Verification items for the finished model (mm, model axes). Face numbers are marked on the shaded views. Give positions to 0.01 mm unless a question says otherwise; leave off trailing zeros. Order: outer loops, then holes, each group sorted by start corner. A loop starts at its lowest first (then second) coordinate and runs counter-clockwise, first axis right, second up.
Autodesk Fusion 360 part; units mm, degrees
sketch "Schizzo1" plane through (0, 0, 0) normal (0, 0, 1) x (1, 0, 0)
  line L0 (50, 150) -> (168.7, 150) construction
  line L1 (168.7, 150) -> (168.7, 89.3) construction
  line L2 (168.7, 89.3) -> (50, 89.3) construction
  line L3 (50, 89.3) -> (50, 150) construction
  line L4 (50, 119.65) -> (168.7, 119.65) construction
  line L5 (109.35, 150) -> (109.35, 89.3) construction
  line L6 (168.6, 89.4) -> (50.1, 89.4)
  line L7 (50.1, 89.4) -> (50.1, 149.9)
  line L8 (50.1, 149.9) -> (168.6, 149.9)
  line L9 (168.6, 149.9) -> (168.6, 89.4)
  line L10 (168.6, 89.4) -> (50.1, 149.9) construction
  line L11 (50.1, 89.4) -> (168.6, 149.9) construction
  point P0 (109.35, 119.65)
  dimension "d1" = 118.7
  dimension "d2" = 60.7
  dimension "d3" = 0.1
  dimension "d4" = 0.1
extrude "Estrusione1" add sketch "Schizzo1" along normal blind 4
fillet "Raccordo1" radius 3 4 edges at (50.1, 89.4, 2) (168.6, 89.4, 2) (50.1, 149.9, 2) (168.6, 149.9, 2)
sketch "Schizzo2" plane through (0, 0, 4) normal (0, 0, 1) x (-1, 0, 0)
  arc A0 (-168.6, -146.9) -> (-165.6, -149.9) centre (-165.6, -146.9) ccw
  line L0 (-165.6, -149.9) -> (-53.1, -149.9)
  arc A1 (-53.1, -149.9) -> (-50.1, -146.9) centre (-53.1, -146.9) ccw
  line L1 (-50.1, -146.9) -> (-50.1, -92.4)
  arc A2 (-50.1, -92.4) -> (-53.1, -89.4) centre (-53.1, -92.4) ccw
  line L2 (-53.1, -89.4) -> (-165.6, -89.4)
  arc A3 (-165.6, -89.4) -> (-168.6, -92.4) centre (-165.6, -92.4) ccw
  line L3 (-168.6, -92.4) -> (-168.6, -146.9)
  line L4 (-50.1, -149.9) -> (-168.6, -149.9) construction
  line L5 (-168.6, -149.9) -> (-168.6, -89.4) construction
  line L6 (-168.6, -89.4) -> (-50.1, -89.4) construction
  line L7 (-50.1, -89.4) -> (-50.1, -149.9) construction
  line L8 (-50.1, -119.65) -> (-168.6, -119.65) construction
  line L9 (-109.35, -149.9) -> (-109.35, -89.4) construction
  line L10 (-166.6, -91.4) -> (-52.1, -91.4)
  line L11 (-52.1, -91.4) -> (-52.1, -147.9)
  line L12 (-52.1, -147.9) -> (-166.6, -147.9)
  line L13 (-166.6, -147.9) -> (-166.6, -91.4)
  line L14 (-166.6, -91.4) -> (-52.1, -147.9) construction
  line L15 (-52.1, -91.4) -> (-166.6, -147.9) construction
  line L16 (-70.6, -91.4) -> (-70.6, -147.9)
  line L17 (-63.6, -147.9) -> (-63.6, -91.4)
  line L18 (-52.1, -121.9) -> (-52.1, -147.9)
  line L19 (-103.6, -147.9) -> (-103.6, -91.4)
  line L20 (-110.6, -147.9) -> (-110.6, -91.4)
  line L21 (-143.6, -147.9) -> (-143.6, -91.4)
  line L22 (-150.6, -147.9) -> (-150.6, -91.4)
  line L23 (-52.1, -91.4) -> (-62.1, -91.4)
  line L24 (-62.1, -91.4) -> (-62.1, -117.4)
  line L25 (-62.1, -117.4) -> (-52.1, -117.4)
  line L26 (-52.1, -117.4) -> (-52.1, -91.4)
  line L27 (-102.1, -117.4) -> (-92.1, -117.4)
  line L28 (-92.1, -117.4) -> (-92.1, -91.4)
  line L29 (-102.1, -91.4) -> (-102.1, -117.4)
  line L30 (-92.1, -91.4) -> (-102.1, -91.4)
  line L31 (-142.1, -117.4) -> (-132.1, -117.4)
  line L32 (-132.1, -117.4) -> (-132.1, -91.4)
  line L33 (-142.1, -91.4) -> (-142.1, -117.4)
  line L34 (-132.1, -91.4) -> (-142.1, -91.4)
  line L35 (-52.1, -117.4) -> (-166.6, -117.4)
  line L36 (-52.1, -121.9) -> (-166.6, -121.9)
  point P0 (-109.35, -119.65)
  point P1 (-109.35, -119.65)
  dimension "d11" = 7
  dimension "d20" = 7
  dimension "d25" = 7
  dimension "d36" = 13.5
  dimension "d37" = 53.5
  dimension "d38" = 93.5
  dimension "d39" = 10
  dimension "d40" = 26
  dimension "d41" = 2
  dimension "d42" = 2
  dimension "d45" = -40
  dimension "d46" = 0
extrude "Estrusione2" cut sketch "Schizzo2" against normal blind 3 contours L10 L13 L22 L35 | L10 L21 L33 L35 | L12 L13 L22 L36 | L10 L31 L32 L33 L34 L35 | L10 L20 L32 L35 | L12 L20 L21 L36 | L10 L19 L29 L35 | L12 L16 L19 L36 | L10 L27 L28 L29 L30 L35 | L10 L16 L28 L35 | L11 L12 L17 L18 L36 | L10 L17 L24 L35 | L10 L11 L23 L24 L25 L26 L35
extrude "Estrusione3" cut sketch "Schizzo2" against normal blind 4 contours L10 L31 L32 L33 L34 L35 | L10 L27 L28 L29 L30 L35 | L10 L11 L23 L24 L25 L26 L35
ref_plane "Piano di lavoro1" through (109.35, 119.65, 4) normal (0, -1, 0) x (1, 0, 0)
sketch "Schizzo3" plane through (0, 119.65, 0) normal (0, -1, 0) x (-1, 0, 0)
  line L0 (-50.1, -4) -> (-168.7, -4) construction
  line L1 (-168.7, -4) -> (-168.7, 0) construction
  line L2 (-168.7, 0) -> (-50.1, 0) construction
  line L3 (-50.1, 0) -> (-50.1, -4) construction
  line L4 (-168.6, -4) -> (-50.1, -4) construction
  line L5 (-50.1, -1) -> (-168.7, -1) construction
  line L6 (-63.6, -4) -> (-63.6, 0) construction
  line L7 (-70.6, -4) -> (-70.6, 0) construction
  line L8 (-63.6, -4) -> (-63.6, -1) construction
  line L9 (-70.6, -4) -> (-70.6, -1) construction
  line L10 (-103.6, -4) -> (-103.6, 0) construction
  line L11 (-110.6, -4) -> (-110.6, 0) construction
  line L12 (-103.6, -4) -> (-103.6, -1) construction
  line L13 (-110.6, -4) -> (-110.6, -1) construction
  line L14 (-143.6, -4) -> (-143.6, 0) construction
  line L15 (-150.6, -4) -> (-150.6, 0) construction
  line L16 (-143.6, -4) -> (-143.6, -1) construction
  line L17 (-150.6, -4) -> (-150.6, -1) construction
  line L18 (-63.6, -4) -> (-65.3321, -1)
  line L19 (-63.6, -4) -> (-60.1359, -4) construction
  line L20 (-70.6, -4) -> (-68.8679, -1)
  line L21 (-70.6, -4) -> (-67.1359, -4) construction
  line L22 (-63.6, -4) -> (-63.6, -1)
  line L23 (-63.6, -1) -> (-65.3321, -1)
  line L24 (-68.8679, -1) -> (-70.6, -1)
  line L25 (-70.6, -1) -> (-70.6, -4)
  line L26 (-103.6, -1) -> (-103.6, -4)
  line L27 (-103.6, -4) -> (-105.3321, -1)
  line L28 (-105.3321, -1) -> (-103.6, -1)
  line L29 (-110.6, -1) -> (-110.6, -4)
  line L30 (-110.6, -4) -> (-108.8679, -1)
  line L31 (-108.8679, -1) -> (-110.6, -1)
  line L32 (-143.6, -1) -> (-143.6, -4)
  line L33 (-143.6, -4) -> (-145.3321, -1)
  line L34 (-145.3321, -1) -> (-143.6, -1)
  line L35 (-150.6, -1) -> (-150.6, -4)
  line L36 (-150.6, -4) -> (-148.8679, -1)
  line L37 (-148.8679, -1) -> (-150.6, -1)
  line L38 (-110.6, -1) -> (-143.6, -1)
  point P0 (-168.7, 0)
  dimension "d28" = 120
  dimension "d29" = 60
  dimension "d30" = 30
  dimension "d31" = 30
  dimension "d32" = 30
  dimension "d33" = 30
extrude "Estrusione4" cut sketch "Schizzo3" along normal blind 25 from surface at 2.5
extrude "Estrusione6" cut sketch "Schizzo3" against normal blind 25 from surface at -2.5
sketch "Schizzo4" plane through (0, 0, 4) normal (0, 0, 1) x (-1, 0, 0)
  line L0 (-50.1, -149.9) -> (-168.6, -149.9) construction
  line L1 (-168.6, -149.9) -> (-168.6, -89.4) construction
  line L2 (-168.6, -89.4) -> (-50.1, -89.4) construction
  line L3 (-50.1, -89.4) -> (-50.1, -149.9) construction
  line L4 (-165.6, -149.9) -> (-53.1, -149.9) construction
  line L5 (-53.1, -89.4) -> (-165.6, -89.4) construction
  line L6 (-50.1, -146.9) -> (-50.1, -92.4) construction
  line L7 (-168.6, -92.4) -> (-168.6, -146.9) construction
  line L8 (-50.1, -149.9) -> (-168.6, -149.9)
  line L9 (-168.6, -149.9) -> (-168.6, -147.9)
  line L10 (-168.6, -147.9) -> (-50.1, -147.9)
  line L11 (-50.1, -147.9) -> (-50.1, -149.9)
  line L12 (-50.1, -89.4) -> (-168.6, -89.4)
  line L13 (-168.6, -89.4) -> (-168.6, -91.4)
  line L14 (-168.6, -91.4) -> (-50.1, -91.4)
  line L15 (-50.1, -91.4) -> (-50.1, -89.4)
  dimension "d51" = 2
  dimension "d52" = 2
extrude "Estrusione5" cut sketch "Schizzo4" against normal blind 2
equation "d28 = 90 deg + 30 deg"
equation "d52 = d51"
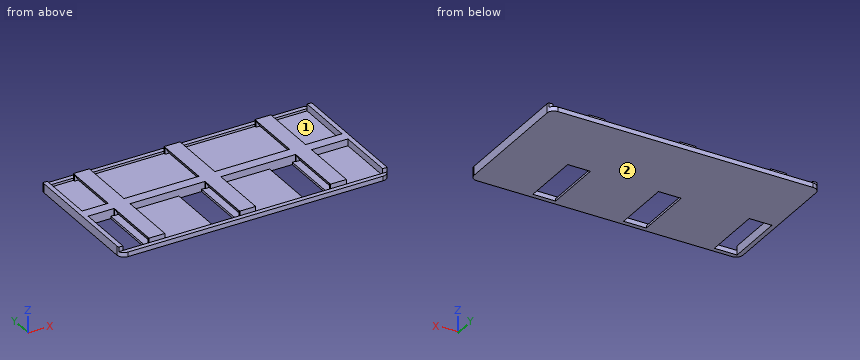
(1) Section check B-B, the plane x = 101. Enter the section's corners in (y, z), then the cut area to 3 significant figures.
Solved:
outline: (89.4, 0) - (91.4, 0) - (91.4, 2) - (89.4, 2) - close; (117.4, 0) - (149.9, 0) - (149.9, 2) - (147.9, 2) - (147.9, 1) - (121.9, 1) - (121.9, 4) - (117.4, 4) - close
area: 52.0 mm2
(2) Scan lines: line 1 (X direction, y = 111, z = 0.35); line 2 (Y direction, x = 70.5, z = 2.6); line 3 (X direction, y = 92, z = 2.1). Record each from-to range of solid material in increasing order.
Solved:
line 1: x = 50.1 to 52.1, 62.1 to 92.1, 102.1 to 132.1, 142.1 to 168.6
line 2: y = 91.4 to 92.15, 117.15 to 122.15, 147.15 to 147.9
line 3: x = 50.13 to 52.1, 63.6 to 70.6, 103.6 to 110.6, 143.6 to 150.6, 166.6 to 168.57
(3) Go/stop test with flat-tipped pins: pin 1 (0.5 mm diameter, centred on x = 150, z = 3, fed in from +Y); pin 2 (1.5 mm diameter, centred on x = 167.5, z = 3.5, fed in from -Y); pin 3 (1.5 mm diameter, centred on x = 62.5, y = 130.5, fed in from +Z). Record where each tip stops, or that it passes through.
Solved:
pin 1: stops at y = 147.9
pin 2: stops at y = 91.4
pin 3: stops at z = 1
(4) Release check for a two-part mould opening along X. For the marked faces 1 and 2 record: pulls with the +X half, pulls with the -X half, needs draft (parallel to the pull), parting line crosses it, or undercut.
Solved:
face 1: undercut
face 2: needs draft
(5) Section check D-D, the plane x = 67. Enter the section's corners in (y, z).
Solved:
outline: (89.4, 0) - (149.9, 0) - (149.9, 2) - (147.9, 2) - (147.9, 4) - (91.4, 4) - (91.4, 2) - (89.4, 2) - close
(6) Section check A-A, the plane y = 115.5. Give the number of separate pieces and of enclosed holes in the cut face, then the cut area to 3 significant figures.
Solved:
separate pieces: 4
enclosed holes: 0
area: 148 mm2
(7) Section check C-C, the plane y = 140. Enter the section's corners in (x, z), then the cut area to 3 significant figures.
Solved:
outline: (50.1, 0) - (168.6, 0) - (168.6, 4) - (166.6, 4) - (166.6, 1) - (148.87, 1) - (150.6, 4) - (143.6, 4) - (145.33, 1) - (108.87, 1) - (110.6, 4) - (103.6, 4) - (105.33, 1) - (68.87, 1) - (70.6, 4) - (63.6, 4) - (65.33, 1) - (52.1, 1) - (52.1, 4) - (50.1, 4) - close
area: 178 mm2
